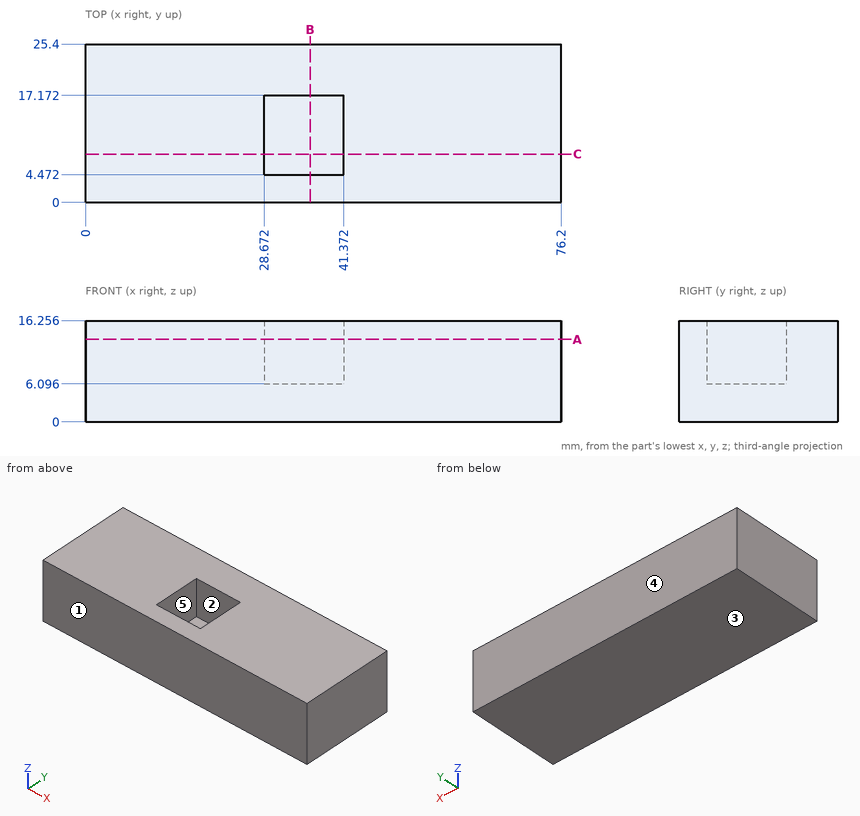
Source: three-view drawing plus pictorial views. Frame: mm from the lowest corner of the part. A direction names the side the tool comes from. Round coordinates to 2 decimals unless told otherwise and drop trailing zeros. Loops run counter-clockwise (first coordinate to the right, second up) from the corner with the lowest first, then second, coordinate; pieces in that order, holes last. Notation, with made-up numbers: M 58.5,66 L 107.5,66 A19 cw 107.5,75 Z; hole C 67,79 d9. An arc over 180 degrees is marked long. Put each result on its own line as item: value.
(1) Section C-C, the plane y = 7.75. Return loops of the section in (x, z), and give its area (3 significant figures).
Solutions:
outline: M 0,0 L 76.2,0 L 76.2,16.26 L 41.37,16.26 L 41.37,6.1 L 28.67,6.1 L 28.67,16.26 L 0,16.26 Z
area: 1,110 mm²
(2) Pull-direction query (Y, two-part tool) for the marked faces 1, 2 and 3; classes: released by +Y, released by -Y, zero draft, split by the parting line, or undercut.
Solutions:
face 1: released by -Y
face 2: undercut
face 3: zero draft
(3) Ray query, line 1 (Y direction, x = 37, z = 6.75); line 2 (X direction, y = 11.75, z = 10); line 3 (Z direction, x = 30.5, y = 10.25). Return the intervals inside material, ascending. Write a range as [from, to].
Solutions:
line 1: [0, 4.47], [17.17, 25.4]
line 2: [0, 28.67], [41.37, 76.2]
line 3: [0, 6.1]
(4) Section B-B, the plane x = 36. Return loops of the section in (y, z), and give its area (3 significant figures).
Solutions:
outline: M 0,0 L 25.4,0 L 25.4,16.26 L 17.17,16.26 L 17.17,6.1 L 4.47,6.1 L 4.47,16.26 L 0,16.26 Z
area: 284 mm²
(5) Section A-A, the plane z = 13.25. Return loops of the section in (x, y).
Solutions:
outline: M 0,0 L 76.2,0 L 76.2,25.4 L 0,25.4 Z; hole M 28.67,4.47 L 41.37,4.47 L 41.37,17.17 L 28.67,17.17 Z
(6) Access query for the marked faces 4 and 5. Directions: +Z, -Z, +X, -X, +Y, -Y. A direction counts if a zero-diameter tool reaches every point of the face in a straight line with its end or side. Return the directions, or none.
Solutions:
face 4: +Z, -Z, +X, -X, +Y
face 5: +Z
(7) First-contact query: pin 1 (6 mm diameter, centred on y = 4, z = 13, fed in from -X); pin 2 (4 mm diameter, centred on x = 37.5, y = 12.5, fed in from +Z). Flat tips, straight axial feed; report the tip coordinate or a pass-through.
Solutions:
pin 1: x = 0
pin 2: z = 6.1
